The model under review builds one solid part; all positions refer to its coordinate system, in mm. A direction names the side the tool comes from. Coordinates: 2 decimals unless noted, no trailing zeros. Write each loop counter-clockwise with the first axis right and the second up, starting at its lowest first coordinate (ties: lowest second). Pieces come first, ordered by that corner, then holes.
1) Machinability: for faces 1 (the cylindrical face through (910, 0, 110)), 2 (the flat face through (464, 0, 0)), 3 (the flat face through (903, -73, 52)), which of the approach directions +Z, -Z, +X, -X, +Y, -Y give a long, thin tool a straight path to every point of the face, cutting with its end or side? Answer none if there is none.
2) Add section A-A, the plane x = 940. State the section outline as (y, z) points, then the cut area to 3 significant figures.
3) For line 1 (X direction, y = 0, z = 108); line 2 (X direction, y = 0, z = 36); line 3 (Y direction, x = 940, z = -18.75), list the stretches that pass through material, from the lowest coordinate up.
4) Add section D-D, the plane x = 478.5. State the section outline as (y, z) points.
5) Add section B-B, the plane y = 73. State the section outline as (x, z) points, then the cut area to 3 significant figures.
6) Add section C-C, the plane y = 0. Give the number of separate pieces and of enclosed holes in the cut face, then the cut area to 3 significant figures.
7) For P1, Ø23, axis at x = 885.5, y = 54.5, coming from the -Z side; P2, Ø10, axis at x = 540.5, z = 81, coming from the +Y side; P3, Ø3, axis at x = 349.5, y = -1, coming from the +Z side, all flat-tipped, find the tip position at first contact; note any pin that passes through.
Autodesk Inventor part; units mm, degrees
ref_plane "YZ Plane" through (0, 0, 0) normal (1, 0, 0) x (0, 1, 0)
ref_plane "XZ Plane" through (0, 0, 0) normal (0, 1, 0) x (-1, 0, 0)
ref_plane "XY Plane" through (0, 0, 0) normal (0, 0, 1) x (1, 0, 0)
sketch "Boceto1" plane through (0, 0, 0) normal (0, 0, 1) x (1, 0, 0)
  circle A0 centre (0, 0) radius 30
  circle A1 centre (0, 0) radius 26.15
  circle A2 centre (940, 0) radius 30
  circle A3 centre (940, 0) radius 26.15
  line L0 (22.3607, -20) -> (917.6393, -20)
  line L1 (26.15, 0) -> (30, 0)
  line L2 (910, 0) -> (940, 0)
  line L3 (22.3607, 20) -> (917.6393, 20)
  dimension "d1" = 52.3
  dimension "d0" = 60
  dimension "d2" = 940
  dimension "d3" = 60
  dimension "d4" = 52.3
extrude "Extrusión1" add sketch "Boceto1" along normal blind 80
sketch "Boceto2" plane through (0, 0, 80) normal (0, 0, 1) x (1, 0, 0)
  arc A0 (22.3607, 20) -> (22.3607, -20) centre (0, 0) ccw
  line L0 (22.3607, -20) -> (917.6393, -20)
  arc A1 (917.6393, -20) -> (917.6393, 20) centre (940, 0) ccw
  line L1 (917.6393, 20) -> (22.3607, 20)
  circle A2 centre (940, 0) radius 26.15
  circle A3 centre (0, 0) radius 26.15
  circle A4 centre (0, 0) radius 30
  circle A5 centre (940, 0) radius 30
  point P0 (917.6393, 20)
  point P1 (22.3607, -20)
extrude "Extrusión2" add sketch "Boceto2" along normal blind 60 contours A4 A0 | A1 A5
sketch "Boceto3" plane through (0, 0, 0) normal (0, 0, -1) x (-1, 0, 0)
  arc A0 (-22.3607, -20) -> (-22.3607, 20) centre (0, 0) ccw
  line L0 (-917.6393, 20) -> (-22.3607, 20)
  arc A1 (-917.6393, 20) -> (-917.6393, -20) centre (-940, 0) ccw
  line L1 (-22.3607, -20) -> (-917.6393, -20)
  circle A2 centre (-940, 0) radius 26.15
  circle A3 centre (0, 0) radius 26.15
  circle A4 centre (0, 0) radius 30
  arc A5 (-917.6393, 20) -> (-917.6393, -20) centre (-940, 0) ccw
  circle A6 centre (-940, 0) radius 30
  point P0 (-22.3607, 20)
extrude "Extrusión3" add sketch "Boceto3" along normal blind 30 contours A4 A0 | A1 A6
sketch "Boceto7" plane through (0, 0, 80) normal (0, 0, 1) x (1, 0, 0)
  line L0 (85, 125) -> (30, 125)
  line L1 (85, 20) -> (85, 125)
  line L2 (33.5, 125) -> (33.5, -125)
  line L3 (30, -125) -> (85, -125)
  line L4 (33.5, 125) -> (85, 125)
  line L5 (85, 125) -> (85, -125)
  line L6 (85, -125) -> (33.5, -125)
  line L7 (33.5, -125) -> (33.5, 125)
  point P0 (0, 0)
extrude "Extrusión7" add sketch "Boceto7" along normal blind 3.5
sketch "Boceto8" plane through (0, 0, 80) normal (0, 0, -1) x (-1, 0, 0)
  line L0 (-33.5, -20) -> (-85, -20)
  line L1 (-85, -125) -> (-85, -20)
  line L2 (-33.5, -125) -> (-85, -125)
  line L3 (-33.5, -20) -> (-33.5, -125)
  line L4 (-85, 20) -> (-33.5, 20)
  line L5 (-33.5, 125) -> (-33.5, 20)
  line L6 (-85, 125) -> (-33.5, 125)
  line L7 (-85, 20) -> (-85, 125)
  line L8 (-33.5, 125) -> (-33.5, -125)
  line L9 (-85, 125) -> (-33.5, 125)
  line L10 (-33.5, -125) -> (-37, -125)
  line L11 (-37, -125) -> (-37, 125)
  line L12 (-37, 125) -> (-33.5, 125)
  line L13 (-33.5, 125) -> (-33.5, -125)
  line L14 (-917.6393, 20) -> (-22.3607, 20)
  line L15 (-470, 20) -> (-470, -237.5428)
  line L16 (-906.5, -20) -> (-855, -20)
  line L17 (-855, -125) -> (-855, -20)
  line L18 (-906.5, -125) -> (-855, -125)
  line L19 (-906.5, -20) -> (-906.5, -125)
  line L20 (-855, 20) -> (-906.5, 20)
  line L21 (-906.5, 125) -> (-906.5, 20)
  line L22 (-855, 125) -> (-906.5, 125)
  line L23 (-855, 20) -> (-855, 125)
  line L24 (-906.5, 125) -> (-906.5, -125)
  line L25 (-855, 125) -> (-906.5, 125)
  line L26 (-906.5, -125) -> (-903, -125)
  line L27 (-903, -125) -> (-903, 125)
  line L28 (-903, 125) -> (-906.5, 125)
  line L29 (-906.5, 125) -> (-906.5, -125)
  line L30 (-855, 125) -> (-903, 125)
  line L31 (-903, 125) -> (-903, -125)
  line L32 (-903, -125) -> (-855, -125)
  line L33 (-855, -125) -> (-855, 125)
  point P0 (0, 0)
  point P1 (-37, 20)
  point P2 (-37, -20)
  point P3 (-903, 20)
  point P4 (-903, -20)
  dimension "d26" = 3.5
extrude "Extrusión8" add sketch "Boceto8" along normal blind 55 contours L3 L2 L11 L0 | L4 L11 L6 L5
fillet "Empalme3" radius 2 2 edges at (37, -72.5, 80) (37, 72.5, 80)
extrude "Extrusión9" add sketch "Boceto8" against normal blind 3.5 contours L33 L16 L27 L14 | L14 L27 L22 L23 | L27 L16 L24 L14 | L14 L21 L22 L27 | L17 L18 L27 L16 | L27 L18 L19 L16
extrude "Extrusión10" add sketch "Boceto8" along normal blind 55 contours L14 L21 L22 L27 | L27 L18 L19 L16
fillet "Empalme4" radius 2 2 edges at (903, -72.5, 80) (903, 72.5, 80)
properties part number "bocina2"
Geometry results:
1. face 1: +Z
1. face 2: -Z, +Y, -Y
1. face 3: -Z, -Y
2. outline: (-30, -30) - (-26.15, -30) - (-26.15, 140) - (-30, 140) - (-30, 0) - close; (26.15, -30) - (30, -30) - (30, 80) - (30, 140) - (26.15, 140) - close
2. area: 1,310 mm2
3. line 1: x = -30 to -26.15, 26.15 to 30, 910 to 913.85, 966.15 to 970
3. line 2: x = -30 to -26.15, 26.15 to 913.85, 966.15 to 970
3. line 3: y = -30 to -26.15, 26.15 to 30
4. outline: (-20, 0) - (20, 0) - (20, 80) - (-20, 80) - close
5. outline: (33.5, 25) - (37, 25) - (37, 78) arc R2 cw to (39, 80) - (85, 80) - (85, 83.5) - (33.5, 83.5) - close; (855, 80) - (901, 80) arc R2 cw to (903, 78) - (903, 25) - (906.5, 25) - (906.5, 83.5) - (855, 83.5) - close
5. area: 747 mm2
6. separate pieces: 3
6. enclosed holes: 0
6. area: 73,400 mm2
7. P1: stops at z = 80
7. P2: stops at y = 20
7. P3: stops at z = 80
